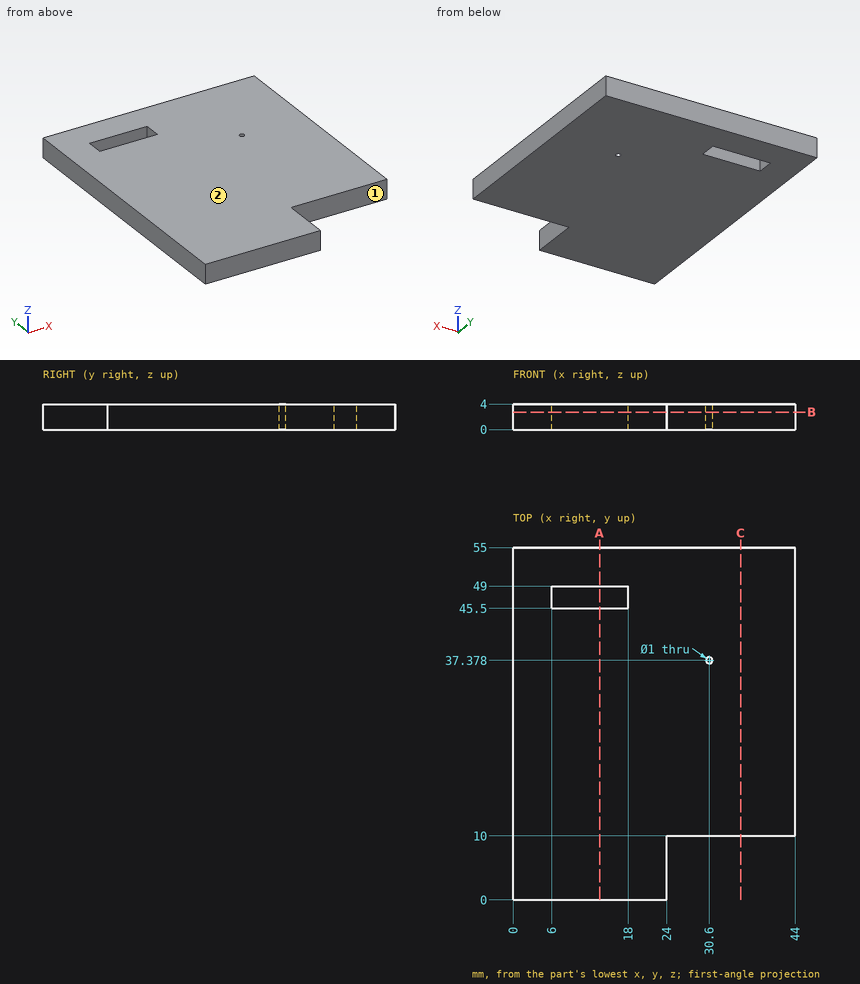
Geometry: see drawing. Coordinates: mm, zero at the bounding-box minimum. A direction names the side the tool comes from. Coordinates: 2 decimals unless noted, no trailing zeros. Write each loop counter-clockwise with the first axis right and the second up, starting at its lowest first coordinate (ties: lowest second). Pieces come first, ordered by that corner, then holes.
1) Section B-B on z = 2.75. Output: boundary loops of the cut face in (x, y).
2) Pin query (flat end, axial travel): pin 1 Ø1.2 at (x, z) = (37, 2) entering from -Y; pin 2 Ø1.2 at (y, z) = (6, 1.5) entering from +X. Return the tip coordinate at first contact, or that it passes through.
3) Section A-A on x = 13.5. Output: boundary loops of the cut face in (y, z), and give its area (3 significant figures).
4) Section C-C on x = 35.5. Output: boundary loops of the cut face in (y, z), and give its area (3 significant figures).
5) Material intervals for line 1 along Y through (x, z) = (30.6, 1.2); line 2 along X through (y, z) = (46.5, 1.3); line 3 along Y through (x, z) = (13.5, 2.4), sorted ascending.
6) Set-up query: the marked faces 1 and 2. Return all of +Z, -Z, +X, -X, +Y, -Y with unobstructed straight access to the full face (end or side cutting, diameter ignored); none if empty.
Check result:
1. outline: (0, 0) - (24, 0) - (24, 10) - (44, 10) - (44, 55) - (0, 55) - close; hole (6, 45.5) - (18, 45.5) - (18, 49) - (6, 49) - close; hole circle Ø1 at (30.6, 37.38)
2. pin 1: stops at y = 10
2. pin 2: stops at x = 24
3. outline: (0, 0) - (45.5, 0) - (45.5, 4) - (0, 4) - close; (49, 0) - (55, 0) - (55, 4) - (49, 4) - close
3. area: 206 mm2
4. outline: (10, 0) - (55, 0) - (55, 4) - (10, 4) - close
4. area: 180 mm2
5. line 1: y = 10 to 36.88, 37.88 to 55
5. line 2: x = 0 to 6, 18 to 44
5. line 3: y = 0 to 45.5, 49 to 55
6. face 1: +Z, -Z, +X, -Y
6. face 2: +Z, +X, -X, +Y, -Y
